Read the model definition and answer for the solid it produces. Units are mm, in the model's axes. Coordinates: 2 decimals unless noted, no trailing zeros. Order: outer loops, then holes, each group sorted by start corner. A loop starts at its lowest first (then second) coordinate and runs counter-clockwise, first axis right, second up. Notation, with made-up numbers: M 23,86 L 52,86 A27 cw 52,111 Z; hole C 44,17.25 d8. An arc over 180 degrees is marked long. Write each question's results on one line, items separated by ' | '.
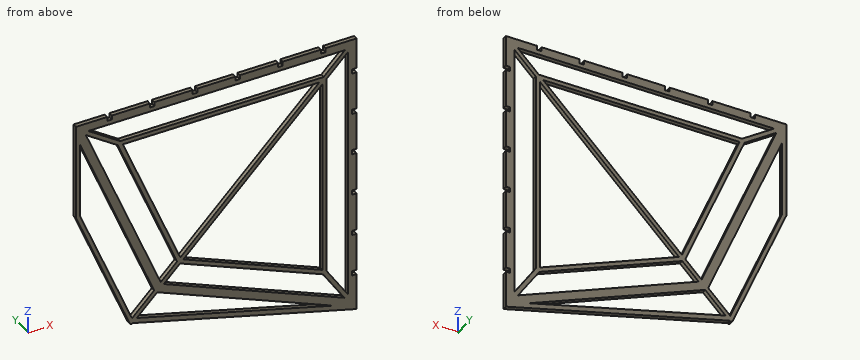
Autodesk Inventor part; units mm, degrees
ref_plane "YZ Plane" through (0, 0, 0) normal (1, 0, 0) x (0, 1, 0)
ref_plane "XZ Plane" through (0, 0, 0) normal (0, 1, 0) x (-1, 0, 0)
ref_plane "XY Plane" through (0, 0, 0) normal (0, 0, 1) x (1, 0, 0)
sketch "草圖1" plane through (0, 0, 0) normal (0, 1, 0) x (-1, 0, 0)
  line L0 (0, 0) -> (0, -200)
  line L1 (0, 0) -> (200, 0)
  line L2 (0, 0) -> (141.4214, -141.4214)
  line L3 (200, 0) -> (141.4214, -141.4214)
  line L4 (141.4214, -141.4214) -> (0, -200)
  line L5 (191.0204, -6) -> (6, -6)
  line L6 (6, -6) -> (6, -191.0204)
  line L7 (6, -191.0204) -> (136.8292, -136.8292)
  line L8 (136.8292, -136.8292) -> (191.0204, -6)
  line L9 (2.1213, 0) -> (142.0427, -139.9214)
  line L10 (0, -2.1213) -> (139.9214, -142.0427)
  line L11 (168.5713, -21) -> (21, -21)
  line L12 (21, -21) -> (21, -168.5713)
  line L13 (21, -168.5713) -> (125.3487, -125.3487)
  line L14 (125.3487, -125.3487) -> (168.5713, -21)
  line L15 (164.0815, -24) -> (24, -24)
  line L16 (24, -24) -> (24, -164.0815)
  line L17 (24, -164.0815) -> (123.0526, -123.0526)
  line L18 (123.0526, -123.0526) -> (164.0815, -24)
  line L19 (191.0204, -6) -> (168.5713, -21)
  line L20 (191.8537, -7.2472) -> (169.4046, -22.2472)
  line L21 (190.187, -4.7528) -> (167.7379, -19.7528)
  line L22 (167.7379, -19.7528) -> (161.3815, -24)
  line L23 (169.4046, -22.2472) -> (163.0482, -26.4944)
  line L24 (24, -164.0815) -> (6, -191.0204)
  line L25 (25.2472, -164.9148) -> (7.2472, -191.8537)
  line L26 (22.7528, -163.2481) -> (4.7528, -190.187)
  line L27 (175, 0) -> (171.8, 0)
  line L28 (171.8, 0) -> (171.8, -3)
  line L29 (171.8, -3) -> (175, -3)
  line L30 (175, -3) -> (175, 0)
  line L31 (141.8, -3) -> (145, -3)
  line L32 (141.8, 0) -> (141.8, -3)
  line L33 (145, -3) -> (145, 0)
  line L34 (111.8, -3) -> (115, -3)
  line L35 (111.8, 0) -> (111.8, -3)
  line L36 (115, -3) -> (115, 0)
  line L37 (81.8, -3) -> (85, -3)
  line L38 (81.8, 0) -> (81.8, -3)
  line L39 (85, -3) -> (85, 0)
  line L40 (51.8, -3) -> (55, -3)
  line L41 (51.8, 0) -> (51.8, -3)
  line L42 (55, -3) -> (55, 0)
  line L43 (21.8, -3) -> (25, -3)
  line L44 (21.8, 0) -> (21.8, -3)
  line L45 (25, -3) -> (25, 0)
  line L46 (0, -200) -> (0, -222)
  line L47 (0, -222) -> (156.9777, -156.9777)
  line L48 (200, 0) -> (222, 0)
  line L49 (141.4214, -141.4214) -> (156.9777, -156.9777)
  line L50 (222, 0) -> (156.9777, -156.9777)
  line L51 (197.0204, 0) -> (197.0204, -60.3062)
  line L52 (0, -222) -> (0, -225)
  line L53 (0, -225) -> (159.099, -159.099)
  line L54 (156.9777, -156.9777) -> (159.099, -159.099)
  line L55 (159.099, -159.099) -> (225, 0)
  line L56 (222, 0) -> (225, 0)
  line L57 (197.0204, -60.3062) -> (197.0204, -67.5488)
  line L58 (0, -200) -> (0, -222)
  line L59 (6, -197.5147) -> (6, -219.5147)
  line L60 (194.0204, -67.5488) -> (194.0204, -14.4361)
  line L61 (142.0427, -139.9214) -> (157.599, -155.4777)
  line L62 (139.9214, -142.0427) -> (157.599, -159.7203)
  line L63 (0, -22) -> (3, -22)
  line L64 (3, -22) -> (3, -25.2)
  line L65 (3, -25.2) -> (0, -25.2)
  line L66 (0, -25.2) -> (0, -22)
  line L67 (3, -52) -> (3, -55.2)
  line L68 (0, -52) -> (3, -52)
  line L69 (3, -55.2) -> (0, -55.2)
  line L70 (3, -82) -> (3, -85.2)
  line L71 (0, -82) -> (3, -82)
  line L72 (3, -85.2) -> (0, -85.2)
  line L73 (3, -112) -> (3, -115.2)
  line L74 (0, -112) -> (3, -112)
  line L75 (3, -115.2) -> (0, -115.2)
  line L76 (3, -142) -> (3, -145.2)
  line L77 (0, -142) -> (3, -142)
  line L78 (3, -145.2) -> (0, -145.2)
  line L79 (3, -172) -> (3, -175.2)
  line L80 (0, -172) -> (3, -172)
  line L81 (3, -175.2) -> (0, -175.2)
  line L82 (155.4777, -157.599) -> (6, -197.5147)
  line L83 (155.7761, -159.5894) -> (8, -199.0507)
  line L84 (8, -199.0507) -> (8, -219.5147)
  line L85 (155.0907, -156.1498) -> (4.5, -196.3627)
  line L86 (4.5, -196.3627) -> (4.5, -219.5147)
  line L87 (155.7761, -159.5894) -> (158.7857, -158.7857)
  line L88 (8, -199.0507) -> (0, -201.187)
  point P0 (8.1213, -6)
  point P1 (137.4505, -135.3292)
  point P2 (135.3292, -137.4505)
  point P3 (6, -8.1213)
  point P4 (121.5526, -123.6739)
  point P5 (24, -26.1213)
  point P6 (21, -23.1213)
  point P7 (123.8487, -125.97)
  point P8 (123.6739, -121.5526)
  point P9 (125.97, -123.8487)
  point P10 (23.1213, -21)
  point P11 (26.1213, -24)
  point P12 (21, -165.8714)
  point P13 (6, -188.3204)
  point P14 (8.4944, -189.9871)
  point P15 (23.4944, -167.5381)
  point P16 (188.3204, -6)
  point P17 (165.8714, -21)
  point P18 (167.5381, -23.4944)
  point P19 (189.9871, -8.4944)
  point P20 (171.8, 0)
  point P21 (141.8, 0)
  point P22 (111.8, 0)
  point P23 (81.8, 0)
  point P24 (51.8, 0)
  point P25 (21.8, 0)
  point P26 (156.9777, -156.9777)
  point P27 (197.0204, -7.1935)
  point P28 (157.5991, -156.7203)
  point P29 (0, -25.2)
  point P30 (0, -55.2)
  point P31 (0, -85.2)
  point P32 (0, -115.2)
  point P33 (0, -145.2)
  point P34 (0, -175.2)
  point P35 (154.2524, -156.3737)
  point P36 (16.5488, -193.1453)
  point P37 (157.1115, -159.2328)
  point P38 (0, -201.187)
  dimension "d0" = 200
  dimension "d1" = 200
  dimension "d2" = 45
  dimension "d3" = 67.5
  dimension "d4" = 6
  dimension "d5" = 1.5
  dimension "d6" = 1.5
  dimension "d9" = 15
  dimension "d10" = 3
  dimension "d11" = 1.5
  dimension "d12" = 1.5
  dimension "d13" = 1.5
  dimension "d14" = 1.5
  dimension "d15" = 3
  dimension "d16" = 3.2
  dimension "d17" = 25
  dimension "d20" = 30
  dimension "d27" = 22
  dimension "d28" = 22
  dimension "d29" = 6
  dimension "d30" = 3
  dimension "d31" = 3
  dimension "d32" = 6
  dimension "d34" = 3
  dimension "d35" = 3
  dimension "d36" = 3.2
  dimension "d37" = 22
  dimension "d40" = 30
  dimension "d49" = 2
  dimension "d50" = 1.5
extrude "擠出1" add sketch "草圖1" along normal blind 3 contours L2 L6 L10 L0 | L1 L9 L5 L2 | L10 L6 L7 L4 L85 L86 L0 L81 L79 L80 L78 L76 L77 L75 L73 L74 L72 L70 L71 L69 L67 L68 L65 L64 L63 | L1 L44 L43 L45 L41 L40 L42 L38 L37 L39 L35 L34 L36 L32 L31 L33 L28 L29 L30 L51 L3 L9 L8 L5 | L5 L9 L11 L2 | L2 L12 L10 L6 | L11 L9 L15 L2 | L2 L16 L10 L12 | L26 L12 L24 L6 | L10 L16 L24 L12 | L5 L19 L11 L22 L21 | L11 L22 L15 L9 | L15 L9 L18 L2 | L2 L17 L10 L16 | L24 L13 L25 L7 | L8 L20 L23 L14 L19 | L11 L14 L23 L18 L15 L22 | L18 L9 L14 L2 | L2 L13 L10 L17 | L24 L17 L10 L13 | L18 L23 L14 L9 | L14 L9 L8 L2 | L2 L7 L10 L13 | L7 L2 L4 L10 | L9 L3 L2 L8 | L4 L49 L47 L62 | L61 L50 L49 L3 | L85 L62 L82 L4 | L4 L86 L85 | L3 L51 L50 L60 | L50 L57 L55 L54 | L54 L87 L62 L47 | L59 L88 L86 L4 | L82 L47 L83 L88 L59 | L62 L87 L83 L47 | L54 L53 L62 L87 | L86 L88 L46 L4
sketch "草圖2" plane through (-3, 0, -25.2) normal (0, 0, 1) x (1, 0, 0)
  line L0 (0, 0) -> (0, 3)
  line L1 (-154.599, 3) -> (-156.099, 3)
  line L2 (0, 0) -> (-3, 0)
  line L3 (-3, 0) -> (-3, 3)
  line L4 (-3, 3) -> (0, 3)
  line L5 (0, 3) -> (0, 0)
  circle A0 centre (-1.5, 1.5) radius 2.1213
  point P0 (3, 0)
  point P1 (3, 3)
  dimension "d45" = 3
  dimension "d46" = 4.2426
sketch "草圖3" plane through (-21.8, 0, -3) normal (-1, 0, 0) x (0, 0, 1)
  line L0 (0, 3) -> (-3, 3)
  line L1 (-3, 3) -> (-3, 0)
  line L2 (-3, 0) -> (0, 0)
  line L3 (0, 0) -> (0, 3)
  circle A0 centre (-1.5, 1.5) radius 2.1213
  point P0 (3, 0)
  dimension "d47" = 4.2426
  dimension "d48" = 1.5
properties part number "side_sail"
(1) Straight lines are drawn through the part: line 1 (X direction, y = 2.85, z = -120.5); line 2 (Z direction, x = -20, y = 0.8); line 3 (Z direction, x = -23.5, y = 0.6). For each, find the intervals that lie inside material, in ascending order.
Conclusion:
line 1: -175.09 to -172.09, -150.09 to -143.59, -127.36 to -124.11, -122.62 to -118.38, -24 to -21, -6 to 0 | line 2: -195.85 to -192.22, -191.72 to -185.22, -172.77 to -167.37, -22.12 to -17.88, -6 to 0 | line 3: -194.91 to -191.29, -190.27 to -183.77, -167.54 to -21, -6 to -3
(2) The part is cut by section C-C, the plane y = 2.05. Count the separate pieces of the cut face and the enclosed holes in it, then the cut area to 3 significant figures.
Conclusion:
separate pieces: 1 | enclosed holes: 8 | area: 7,220 mm²
(3) The part is cut by section B-B, the plane x = -32. Write down the section's boundary in (y, z), then the cut area to 3 significant figures.
Conclusion:
outline: M 0,-192.64 L 3,-192.64 L 3,-189.02 L 0,-189.02 Z; M 0,-186.75 L 3,-186.75 L 3,-180.25 L 0,-180.25 Z; M 0,-164.01 L 3,-164.01 L 3,-160.77 L 0,-160.77 Z; M 0,-34.12 L 3,-34.12 L 3,-29.88 L 0,-29.88 Z; M 0,-24 L 3,-24 L 3,-21 L 0,-21 Z; M 0,-6 L 3,-6 L 3,0 L 0,0 Z | area: 79.8 mm²
(4) Given pin 1 (1.5 mm diameter, centred on x = -2, y = 1, fed in from +Z); pin 2 (0.9 mm diameter, centred on x = -1, y = 2, fed in from -Z); pin 3 (0.9 mm diameter, centred on x = -114, y = 2, fed in from +Z); pin 4 (0.9 mm diameter, centred on x = -2, y = 1.5, fed in from -Z), each flat-ended and moving along its own axis, determine where each tip first touches the part or whether it passes through.
Conclusion:
pin 1: z = 0 | pin 2: z = -201.04 | pin 3: z = -3 | pin 4: z = -200.77
(5) The part is cut by section A-A, the plane z = -102. Write down the section's boundary in (x, y).
Conclusion:
outline: M -182.75,0 L -179.75,0 L -179.75,3 L -182.75,3 Z; M -157.75,0 L -151.26,0 L -151.26,3 L -157.75,3 Z; M -135.02,0 L -131.77,0 L -131.77,3 L -135.02,3 Z; M -104.12,0 L -99.88,0 L -99.88,3 L -104.12,3 Z; M -24,0 L -21,0 L -21,3 L -24,3 Z; M -6,0 L 0,0 L 0,3 L -6,3 Z
